```python
from build123d import *

# Parameters (mm, degrees)
SKETCH1_R           = 2
BOSS_EXTRUDE1_DEPTH = 304.65
CUT_EXTRUDE1_START  = -20
CUT_EXTRUDE1_DEPTH  = 20
CUT_EXTRUDE2_START  = -304.65
SKETCH4_R           = 2
CUT_EXTRUDE2_DEPTH  = 304.65


# Read off the part's stored shape, not the designer's step: Cut-Extrude1
with BuildPart() as part:
    # Sketch1 → Boss-Extrude1 (new, symmetric)
    with BuildSketch(Plane.XY):
        Polygon((10, 10), (10, 4.610379336), (8.2, 3.1), (8.2, 5.5), (6.560660172, 5.5), (3.9, 2.839339828), (3.9, 0.519615242), (3.6, 0), (3.9, -0.519615242), (3.9, -2.839339828), (6.560660172, -5.5), (8.2, -5.5), (8.2, -3.1), (10, -4.610379336), (10, -10), (4.610379336, -10), (3.1, -8.2), (5.5, -8.2), (5.5, -6.560660172), (2.839339828, -3.9), (0.519615242, -3.9), (0, -3.6), (-0.519615242, -3.9), (-2.839339828, -3.9), (-5.5, -6.560660172), (-5.5, -8.2), (-3.1, -8.2), (-4.610379336, -10), (-10, -10), (-10, -4.610379336), (-8.2, -3.1), (-8.2, -5.5), (-6.560660172, -5.5), (-3.9, -2.839339828), (-3.9, -0.519615242), (-3.6, 0), (-3.9, 0.519615242), (-3.9, 2.839339828), (-6.560660172, 5.5), (-8.2, 5.5), (-8.2, 3.1), (-10, 4.610379336), (-10, 10), (-4.610379336, 10), (-3.1, 8.2), (-5.5, 8.2), (-5.5, 6.560660172), (-2.839339828, 3.9), (-0.519615242, 3.9), (0, 3.6), (0.519615242, 3.9), (2.839339828, 3.9), (5.5, 6.560660172), (5.5, 8.2), (3.1, 8.2), (4.610379336, 10), align=None)
        with Locations(Location((0, 0, 0), (0, 0, 180))):
            Circle(SKETCH1_R, mode=Mode.SUBTRACT)
    extrude(amount=BOSS_EXTRUDE1_DEPTH, both=True)

    # Cut-Extrude1 outline → Cut-Extrude1 (cut)
    with BuildSketch(Plane(origin=(10, 0, 0), x_dir=(0, 0, -1), z_dir=(1, 0, 0)).offset(CUT_EXTRUDE1_START)):
        with BuildLine():
            Line((272.469540788, -4.610379336), (276.830459212, -4.610379336))
            ThreePointArc((276.830459212, -4.610379336), (279.606428288, -1.201590041), (278.699691346, 3.1))
            ThreePointArc((278.699691346, 3.1), (274.65, 5.1), (270.600308654, 3.1))
            ThreePointArc((270.600308654, 3.1), (269.693571712, -1.201590041), (272.469540788, -4.610379336))
        make_face()
    extrude(amount=CUT_EXTRUDE1_DEPTH, mode=Mode.SUBTRACT)

    # Sketch4 → Cut-Extrude2 (cut)
    with BuildSketch(Plane.XY.offset(304.65).offset(CUT_EXTRUDE2_START)):
        Polygon((-5.5, 6.560660172), (-5.5, 8.2), (-3.1, 8.2), (-4.610379336, 10), (-10, 10), (-10, 4.610379336), (-8.2, 3.1), (-8.2, 5.5), (-6.560660172, 5.5), (-3.9, 2.839339828), (-3.9, 0.519615242), (-3.6, 0), (-3.9, -0.519615242), (-3.9, -2.839339828), (-6.560660172, -5.5), (-8.2, -5.5), (-8.2, -3.1), (-10, -4.610379336), (-10, -10), (-4.610379336, -10), (-3.1, -8.2), (-5.5, -8.2), (-5.5, -6.560660172), (-2.839339828, -3.9), (-0.519615242, -3.9), (0, -3.6), (0.519615242, -3.9), (2.839339828, -3.9), (5.5, -6.560660172), (5.5, -8.2), (3.1, -8.2), (4.610379336, -10), (10, -10), (10, -4.610379336), (8.2, -3.1), (8.2, -5.5), (6.560660172, -5.5), (3.9, -2.839339828), (3.9, -0.519615242), (3.6, 0), (3.9, 0.519615242), (3.9, 2.839339828), (6.560660172, 5.5), (8.2, 5.5), (8.2, 3.1), (10, 4.610379336), (10, 10), (4.610379336, 10), (3.1, 8.2), (5.5, 8.2), (5.5, 6.560660172), (2.839339828, 3.9), (0.519615242, 3.9), (0, 3.6), (-0.519615242, 3.9), (-2.839339828, 3.9), align=None)
        with Locations(Location((0, 0, 0), (0, 0, 180))):
            Circle(SKETCH4_R, mode=Mode.SUBTRACT)
    extrude(amount=CUT_EXTRUDE2_DEPTH, mode=Mode.SUBTRACT)


solid = part.part
```
Verification items for the finished model (mm, model axes). Give positions to 0.01 mm unless a question says otherwise; leave off trailing zeros. Return JSON: item names as keys, results as strings. Group by question number.
1) Go/stop test with flat-tipped pins: pin 1 Ø2.5 at (x, z) = (2, -296.5) entering from -Y; pin 2 Ø1.2 at (y, z) = (-1.5, -81) entering from +X; pin 3 Ø3 at (y, z) = (2.5, -223.5) entering from +X. Record where each tip stops, or that it passes through.
2) Mould release check, pull along X, two halves, no side actions. Record for faces 1 (the face through (10, -7, -150)), 2 (the face through (-10, -7, -150)), 3 (the face through (0.1, 2.4, -304.65)): pulls with the +X half, pulls with the -X half, needs draft (parallel to the pull), parting line crosses it, or undercut.
3) Scan lines: line 1 (Y direction, x = 0, z = -284.75); line 2 (X direction, y = 3.5, z = -187); line 3 (X direction, y = -6.5, z = -232.5). Record each from-to range of solid material in increasing order.
Answer block:
{
 "1": {"pin 1": "stops at y = -8.38", "pin 2": "stops at x = 3.9", "pin 3": "stops at x = 9.27"},
 "2": {"face 1": "pulls with the +X half", "face 2": "pulls with the -X half", "face 3": "needs draft"},
 "3": {"line 1": "y = -3.6 to -2, 2 to 3.6", "line 2": "x = -8.68 to -8.2, -4.56 to 4.56, 8.2 to 8.68", "line 3": "x = -10 to -5.44, 5.44 to 10"}
}
